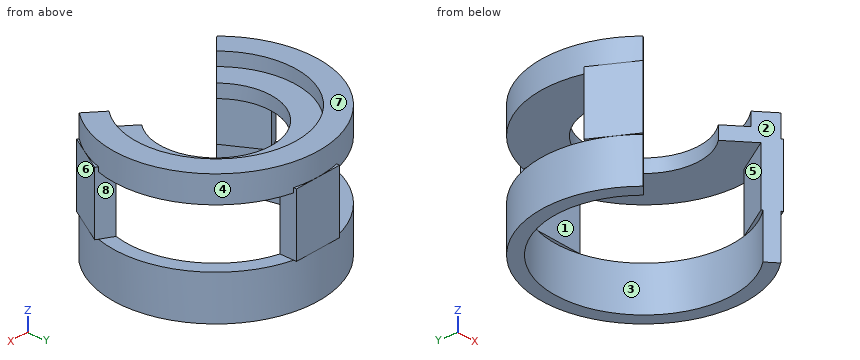
```python
from build123d import *

# Parameters (mm, degrees)
F0_R      = 23
F0_R_2    = 20
F1_DEPTH  = 10
F3_R      = 23
F3_R_2    = 18
F4_DEPTH  = 6
F5_R      = 23
F5_R_2    = 12.5
F6_DEPTH  = 3
F7_W      = 10.728056
F7_H      = 3.725031
F8_DEPTH  = 14
F10_DEPTH = 20


with BuildPart() as f1:
    # F0 (on Top) → F1 (new body)
    with BuildSketch(Plane.XY):
        Circle(F0_R)
        Circle(F0_R_2, mode=Mode.SUBTRACT)
    extrude(amount=-F1_DEPTH)



with BuildPart() as f4:
    # F3 (on offset) → F4 (new body)
    with BuildSketch(Plane.XY.offset(13)):
        Circle(F3_R)
        Circle(F3_R_2, mode=Mode.SUBTRACT)
    extrude(amount=F4_DEPTH)


with BuildPart() as f6:
    # F5 (on offset) → F6 (new body)
    with BuildSketch(Plane.XY.offset(13)):
        Circle(F5_R)
        Circle(F5_R_2, mode=Mode.SUBTRACT)
    extrude(amount=F6_DEPTH)


with BuildPart() as f1_1:
    add(f1.part)

    add(f4.part)  # F8 merges F4

    add(f6.part)  # F8 merges F6
    # F7 (on Top) → F8 (join)
    with BuildSketch(Plane.XY):
        with Locations((-0.054133, 21.146403)):
            Rectangle(F7_W, F7_H)
        Polygon((-22.581255, -6.905955), (-17.217227, -16.196724), (-13.991256, -14.334209), (-19.355284, -5.043439), align=None)
        Polygon((17.27136, -16.102963), (22.635388, -6.812194), (19.409416, -4.949678), (14.045388, -14.240448), align=None)
    extrude(amount=F8_DEPTH)


with BuildPart() as f10:
    # F9 (on Top) → F10 (new body, symmetric)
    with BuildSketch(Plane.XY):
        Polygon((20.578749, -18.006055), (0, 0), (-19.199688, -17.210485), (0.803183, -30.16689), align=None)
    extrude(amount=F10_DEPTH, both=True)


with BuildPart() as f1_2:
    add(f1_1.part)

    # F11: cut F10
    add(f10.part, mode=Mode.SUBTRACT)


solid = f1_2.part
```
Could you check a few things on this model? Use its own coordinates, in mm. Face numbers are marked on the shaded views. A direction names the side the tool comes from. Coordinates: 2 decimals unless noted, no trailing zeros. Write each loop counter-clockwise with the first axis right and the second up, starting at its lowest first coordinate (ties: lowest second). Pieces come first, ordered by that corner, then holes. Notation, with made-up numbers: (35.25, 42) - (47.25, 42) arc R21 ccw to (47.25, 61) - close; hole circle Ø9 at (-17.5, 72.5). An arc over 180 degrees is marked (long way). Use a Markdown table: item, result.
Q1. Thinking about a two-plate mould opening in Z: for the marked faces 6, 7 and 8, which applies, +Z half, -Z half, draft (parallel to the pull), parting line (faces both ways), or undercut?
Geometry check:
| item | result |
|---|---|
| face 6 | draft |
| face 7 | +Z half |
| face 8 | undercut |
Q2. Which directions (+Z, -Z, +X, -X, +Y, -Y) give clear straight access to the entire face, cutting with the end or side of a thin tool? Please do the marked faces 1, 2, 3, 4 and 5.
Geometry check:
| item | result |
|---|---|
| face 1 | -Z, +X, -X, -Y |
| face 2 | +Z, -Z, -Y |
| face 3 | -Z |
| face 4 | +Z |
| face 5 | -Z, +Y |
Q3. I'm going to push flat-ended pins straight in: pin 1 Ø2 at (x, y) = (-15, 10.5) entering from -Z; pin 2 Ø4 at (y, z) = (21.5, 4) entering from -X; pin 3 Ø1 at (x, y) = (-6.5, 13.5) entering from +Z. Where does each tip first touch, or does it pass through?
Geometry check:
| item | result |
|---|---|
| pin 1 | stops at z = 13 |
| pin 2 | stops at x = -5.42 |
| pin 3 | stops at z = 16 |
Q4. Imagine slicing it at B-B (y = 0). List the corners of the cut face in (x, z) for me.
Geometry check:
| item | result |
|---|---|
| outline | (-23, -10) - (-20, -10) - (-20, 0) - (-23, 0) - close; (-23, 13) - (-12.5, 13) - (-12.5, 16) - (-18, 16) - (-18, 19) - (-23, 19) - close; (12.5, 13) - (23, 13) - (23, 19) - (18, 19) - (18, 16) - (12.5, 16) - close; (20, -10) - (23, -10) - (23, 0) - (20, 0) - close |
Q5. Imagine slicing it at A-A (z = 2.75). List the corners of the cut face in (x, y) for me.
Geometry check:
| item | result |
|---|---|
| outline | (-22.58, -6.91) - (-17.51, -15.69) - (-14.67, -13.15) - (-19.36, -5.04) - close; (-5.42, 19.28) - (5.31, 19.28) - (5.31, 23.01) - (-5.42, 23.01) - close; (14.79, -12.94) - (17.65, -15.44) - (22.64, -6.81) - (19.41, -4.95) - close |
Q6. Please list where these lines run through material, in increasing order: L1, parallel to X at y = 0, z = 17.7; L2, parallel to Y at x = 0, z = -7.25; L3, parallel to Y at x = 0, z = 17.65.
Geometry check:
| item | result |
|---|---|
| L1 | x = -23 to -18, 18 to 23 |
| L2 | y = 20 to 23 |
| L3 | y = 18 to 23 |
Q7. Imagine slicing it at D-D (y = -9). List the corners of the cut face in (x, z) for me.
Geometry check:
| item | result |
|---|---|
| outline | (-21.37, 0) - (-21.17, 0) - (-21.17, -10) - (-17.86, -10) - (-17.86, 0) - (-17.07, 0) - (-17.07, 13) - (-10.04, 13) - (-10.04, 16) - (-15.59, 16) - (-15.59, 19) - (-21.17, 19) - (-21.17, 14) - (-21.37, 14) - close; (10.29, 13) - (17.07, 13) - (17.07, 0) - (17.86, 0) - (17.86, -10) - (21.17, -10) - (21.17, 0) - (21.37, 0) - (21.37, 14) - (21.17, 14) - (21.17, 19) - (15.59, 19) - (15.59, 16) - (10.29, 16) - close |
